```python
from build123d import *

# Parameters (mm, degrees)
SKETCH1_W           = 23
SKETCH1_H           = 20
BOSS_EXTRUDE1_DEPTH = 3
SKETCH2_W           = 20
SKETCH2_H           = 37
BOSS_EXTRUDE2_DEPTH = 2.7
SKETCH3_W           = 20
SKETCH3_H           = 37
BOSS_EXTRUDE3_DEPTH = 2.7
SKETCH4_W           = 28.4
SKETCH4_H           = 8
BOSS_EXTRUDE4_DEPTH = 3
SKETCH5_W           = 28.4
SKETCH5_H           = 47
BOSS_EXTRUDE5_DEPTH = 3
SKETCH6_W           = 5
SKETCH6_H           = 15
BOSS_EXTRUDE6_DEPTH = 20
SKETCH7_W           = 5
SKETCH7_H           = 15
BOSS_EXTRUDE7_DEPTH = 20
SKETCH8_W           = 8
SKETCH8_H           = 8
CUT_EXTRUDE1_DEPTH  = 15
SKETCH9_R           = 3
CUT_EXTRUDE2_DEPTH  = 15
SKETCH10_W          = 28.45
SKETCH10_H          = 26
CUT_EXTRUDE3_DEPTH  = 1.5
SKETCH12_W          = 23
SKETCH12_H          = 1.5
CUT_EXTRUDE4_DEPTH  = 15
SKETCH13_W          = 28.4
SKETCH13_H          = 10.836340194
BOSS_EXTRUDE8_DEPTH = 2


with BuildPart() as part:
    # Sketch1 → Boss-Extrude1 (new body)
    with BuildSketch(Plane(origin=(0, 0, 0), x_dir=(1, 0, 0), z_dir=(0, 1, 0))):
        with Locations((11.5, 10)):
            Rectangle(SKETCH1_W, SKETCH1_H)
    extrude(amount=BOSS_EXTRUDE1_DEPTH)

    # Sketch2 → Boss-Extrude2 (add)
    with BuildSketch(Plane.ZY):
        with Locations((-10, 18.5)):
            Rectangle(SKETCH2_W, SKETCH2_H)
    extrude(amount=BOSS_EXTRUDE2_DEPTH)

    # Sketch3 → Boss-Extrude3 (add)
    with BuildSketch(Plane(origin=(23, 0, 0), x_dir=(0, 0, -1), z_dir=(1, 0, 0))):
        with Locations((10, 18.5)):
            Rectangle(SKETCH3_W, SKETCH3_H)
    extrude(amount=BOSS_EXTRUDE3_DEPTH)

    # Sketch4 → Boss-Extrude4 (add)
    with BuildSketch(Plane.XY):
        with Locations((11.5, 4)):
            Rectangle(SKETCH4_W, SKETCH4_H)
    extrude(amount=BOSS_EXTRUDE4_DEPTH)

    # Sketch5 → Boss-Extrude5 (add)
    with BuildSketch(Plane(origin=(0, 0, -20), x_dir=(-1, 0, 0), z_dir=(0, 0, -1))):
        with Locations((-11.5, 23.5)):
            Rectangle(SKETCH5_W, SKETCH5_H)
    extrude(amount=BOSS_EXTRUDE5_DEPTH)

    # Sketch6 → Boss-Extrude6 (add)
    with BuildSketch(Plane(origin=(25.7, 0, 0), x_dir=(0, 0, -1), z_dir=(1, 0, 0))):
        with Locations((20.5, 39.5)):
            Rectangle(SKETCH6_W, SKETCH6_H)
    extrude(amount=BOSS_EXTRUDE6_DEPTH)

    # Sketch7 → Boss-Extrude7 (add)
    with BuildSketch(Plane.ZY.offset(2.7)):
        with Locations((-20.5, 39.5)):
            Rectangle(SKETCH7_W, SKETCH7_H)
    extrude(amount=BOSS_EXTRUDE7_DEPTH)

    # Sketch8 → Cut-Extrude1 (cut)
    with BuildSketch(Plane(origin=(0, 3, 0), x_dir=(1, 0, 0), z_dir=(0, 1, 0))):
        with Locations((11.5, 10)):
            Rectangle(SKETCH8_W, SKETCH8_H)
    extrude(amount=-CUT_EXTRUDE1_DEPTH, mode=Mode.SUBTRACT)

    # Sketch9 → Cut-Extrude2 (cut)
    with BuildSketch(Plane.XY.offset(-18)):
        with Locations((-12.7, 39)):
            Circle(SKETCH9_R)
        with Locations((35.7, 39)):
            Circle(SKETCH9_R)
    extrude(amount=-CUT_EXTRUDE2_DEPTH, mode=Mode.SUBTRACT)

    # Sketch10 → Cut-Extrude3 (cut)
    with BuildSketch(Plane.XZ):
        with Locations((11.525, -10)):
            Rectangle(SKETCH10_W, SKETCH10_H)
    extrude(amount=-CUT_EXTRUDE3_DEPTH, mode=Mode.SUBTRACT)

    # Sketch12 → Cut-Extrude4 (cut)
    with BuildSketch(Plane(origin=(0, 47, 0), x_dir=(1, 0, 0), z_dir=(0, 1, 0))):
        with Locations((11.5, 20.75)):
            Rectangle(SKETCH12_W, SKETCH12_H)
    extrude(amount=-CUT_EXTRUDE4_DEPTH, mode=Mode.SUBTRACT)

    # Sketch13 → Boss-Extrude8 (add)
    with BuildSketch(Plane.XY):
        with Locations((11.5, 31.581829903)):
            Rectangle(SKETCH13_W, SKETCH13_H)
    extrude(amount=BOSS_EXTRUDE8_DEPTH)


solid = part.part
```
Here's how the part is built. I have some questions about the finished solid (model axes, mm). A direction names the side the tool comes from. Coordinates: 2 decimals unless noted, no trailing zeros. Order: outer loops, then holes, each group sorted by start corner. A loop starts at its lowest first (then second) coordinate and runs counter-clockwise, first axis right, second up. Notation, with made-up numbers: (-14, 45.25) - (14, 45.25) arc R13 ccw to (14, 69.25) - close; hole circle Ø7 at (85, 49.25). An arc over 180 degrees is marked (long way). One line per question, with ' | ' between items.
(1) Suppose I cut it at B-B on x = 3. List the corners of the cut face in (y, z) for me.
Report:
outline: (1.5, -23) - (47, -23) - (47, -21.5) - (32, -21.5) - (32, -20) - (3, -20) - (3, 0) - (8, 0) - (8, 3) - (1.5, 3) - close; (26.16, 0) - (37, 0) - (37, 2) - (26.16, 2) - close
(2) If we mould it in two halves opening along X, with no side actions, what happens to faces 1 (the flat face through (11, 6, 0)), 2 (the flat face through (45.7, 40, -20)), 3 (the flat face through (36, 32, -20))? For each: pulls with the +X half, pulls with the -X half, needs draft (parallel to the pull), parting line crosses it, or undercut.
Report:
face 1: undercut | face 2: pulls with the +X half | face 3: needs draft
(3) Suppose I cut it at D-D on z = -17. List the corners of the cut face in (x, y) for me.
Report:
outline: (-2.7, 1.5) - (25.7, 1.5) - (25.7, 37) - (23, 37) - (23, 3) - (0, 3) - (0, 37) - (-2.7, 37) - close
(4) Suppose I cut it at A-A on z = -9. List the corners of the cut face in (x, y) for me, and give its area (3 significant figures).
Report:
outline: (-2.7, 1.5) - (7.5, 1.5) - (7.5, 3) - (0, 3) - (0, 37) - (-2.7, 37) - close; (15.5, 1.5) - (25.7, 1.5) - (25.7, 37) - (23, 37) - (23, 3) - (15.5, 3) - close | area: 214 mm2
(5) Will these pins go through, and if not, where does the flat tip stop? pin 1 (10 mm diameter, centred on x = 12, z = -12, fed in from +Y); pin 2 (5 mm diameter, centred on y = 11.5, z = -12.5, fed in from +X); pin 3 (3 mm diameter, centred on x = 24.5, y = 44.5, fed in from +Z).
Report:
pin 1: stops at y = 3 | pin 2: stops at x = 25.7 | pin 3: stops at z = -18
(6) Suppose I cut it at C-C on y = 39. List the corners of the cut face in (x, z) for me, and give its area (3 significant figures).
Report:
outline: (-22.7, -23) - (-15.7, -23) - (-15.7, -18) - (-22.7, -18) - close; (-9.7, -23) - (32.7, -23) - (32.7, -18) - (25.7, -18) - (25.7, -20) - (23, -20) - (23, -21.5) - (0, -21.5) - (0, -20) - (-2.7, -20) - (-2.7, -18) - (-9.7, -18) - close; (38.7, -23) - (45.7, -23) - (45.7, -18) - (38.7, -18) - close | area: 191 mm2
(7) For faces 4 (the flat face through (24, 42, -20)), 5 (the flat face through (12, 18, -20)), 6 (the flat face through (11, 2, -6)), which set-ups out of +Z, -Z, +X, -X, +Y, -Y let a thin tool reach every point of the face, with its end or its side?
Report:
face 4: +Z, +Y | face 5: +Y | face 6: +Y, -Y
(8) If I drill on L1, parallel to X at y = 8, z = -11.5; L2, parallel to Y at x = 35.7, z = -19.25; L3, parallel to Y at x = 16.5, z = -5, over which ranges is the centre line in solid material (lowest first)?
Report:
L1: x = -2.7 to 0, 23 to 25.7 | L2: y = 32 to 36, 42 to 47 | L3: y = 1.5 to 3
